Can you work these out from the model? Positions are in its coordinate system, mm. A direction names the side the tool comes from. Round coordinates to 2 decimals unless told otherwise and drop trailing zeros. Write each loop counter-clockwise with the first axis right and the second up, starting at its lowest first coordinate (ties: lowest second). Pieces come first, ordered by that corner, then holes. Notation, with made-up numbers: (46, 44.5) -> (73, 44.5) arc R12 ccw to (73, 65.5) -> close; hole circle Ø10 at (26.25, 47). An arc over 180 degrees is marked (long way). Write item = value, one per line. Start each with the question number.
1) Imagine slicing it at A-A, the plane z = 9.25. Please give me the cut outline in (x, y).
2) Imagine slicing it at B-B, the plane x = -7.5. Please give me the cut outline in (y, z).
3) Thinking about a two-plate mould opening in Y: for faces 1 (the face through (-11.356, -23.102, 3.143)), 2 (the face through (-14.274, 0.628, 5.899)), 3 (the face through (9.23, -0.57, 13.11)), 4 (the face through (11, 6, 6.35)), which applies, +Y half, -Y half, draft (parallel to the pull), parting line (faces both ways), or undercut?
4) I'm going to push flat-ended pins straight in: pin 1 (6.5 mm diameter, centred on x = 23.81, y = 0, fed in from -Z); pin 2 (8 mm diameter, centred on y = -1.5, z = 9.5, fed in from +X); pin 3 (23 mm diameter, centred on x = 1.5, y = 3.5, fed in from +Z); pin 4 (1 mm diameter, centred on x = -14.5, y = 0.5, fed in from +Z). Where does each tip first touch, or does it pass through?
5) Imagine slicing it at C-C, the plane y = -19.5. Please give me the cut outline in (x, z).
6) If I drill on line 1 (Z direction, x = 0, y = -21); line 2 (Y direction, x = -4.5, z = 10.5); line 3 (X direction, y = 3.5, z = 1), over which ranges is the centre line in solid material (lowest first)?
7) Imagine slicing it at D-D, the plane z = 4. State how many separate pieces and enclosed holes the cut face has, then the cut area to 3 significant figures.
8) For faces 5 (the face through (-13, 7, 5.461)), 6 (the face through (-7, 0, 0)), 7 (the face through (-5, 5, 25.4)), 8 (the face through (-6.35, -1, 13)), 9 (the face through (-14.274, 0.628, 0.438)), which set-ups out of +Z, -Z, +X, -X, +Y, -Y let a thin tool reach every point of the face, with its end or its side?
from build123d import *

# Parameters (mm, degrees)
SKETCH1_R              = 14.2875
BOSS_EXTRUDE1_DEPTH    = 0.889
SKETCH2_R              = 28.575
BOSS_EXTRUDE2_DEPTH    = 4.572
SKETCH3_R              = 14.2875
BOSS_EXTRUDE3_DEPTH    = 0.889
SKETCH4_R              = 12.192
BOSS_EXTRUDE4_DEPTH    = 19.05
SKETCH5_R              = 2.54
CUT_EXTRUDE1_DEPTH     = 48.2636263
CUT_EXTRUDE2_DEPTH     = 48.730716001
F_10_24_TAPPED_HOLE1_D = 3.7973
CIRPATTERN1_COUNT      = 2
CIRPATTERN1_ANGLE      = 90


with BuildPart() as part:
    # Sketch1 → Boss-Extrude1 (new body)
    with BuildSketch(Plane.XY):
        Circle(SKETCH1_R)
    extrude(amount=BOSS_EXTRUDE1_DEPTH)

    # Sketch2 → Boss-Extrude2 (add)
    with BuildSketch(Plane.XY.offset(0.889)):
        Circle(SKETCH2_R)
    extrude(amount=BOSS_EXTRUDE2_DEPTH)

    # Sketch3 → Boss-Extrude3 (add)
    with BuildSketch(Plane.XY.offset(5.461)):
        Circle(SKETCH3_R)
    extrude(amount=BOSS_EXTRUDE3_DEPTH)

    # Sketch4 → Boss-Extrude4 (add)
    with BuildSketch(Plane.XY.offset(6.35)):
        with Locations(Location((0, 0, 0), (0, 0, 180))):
            Circle(SKETCH4_R)
    extrude(amount=BOSS_EXTRUDE4_DEPTH)

    # Sketch5 → Cut-Extrude1 (cut, through all)
    with BuildSketch(Plane(origin=(0, 0, 0.889), x_dir=(-1, 0, 0), z_dir=(0, 0, -1))):
        with Locations((-11.90625, 20.622229928)):
            Circle(SKETCH5_R)
        with Locations((11.90625, 20.622229928)):
            Circle(SKETCH5_R)
        with Locations((23.8125, 0)):
            Circle(SKETCH5_R)
        with Locations((11.90625, -20.622229928)):
            Circle(SKETCH5_R)
        with Locations((-11.90625, -20.622229928)):
            Circle(SKETCH5_R)
        with Locations((-23.8125, 0)):
            Circle(SKETCH5_R)
    extrude(amount=-CUT_EXTRUDE1_DEPTH, mode=Mode.SUBTRACT)

    # Sketch6 → Cut-Extrude2 (cut, through all)
    with BuildSketch(Plane.XY.offset(25.4)):
        Polygon((0, 7.332348419), (-6.35, 3.666174209), (-6.35, -3.666174209), (0, -7.332348419), (6.35, -3.666174209), (6.35, 3.666174209), align=None)
    extrude(amount=-CUT_EXTRUDE2_DEPTH, mode=Mode.SUBTRACT)

    # #10-24 Tapped Hole1 (through all)
    with Locations(Plane(origin=(12.192, 0, 14.9225), x_dir=(0, 0, 1), z_dir=(1, 0, 0))):
        with Locations((0, 0)):
            f_10_24_tapped_hole1 = Hole(F_10_24_TAPPED_HOLE1_D / 2)

    # CirPattern1: #10-24 Tapped Hole1 ×2 about axis
    cirpattern1_axis = Axis((0, 0, 5.461), (0, 0, 1))
    for i in range(1, CIRPATTERN1_COUNT):
        add(f_10_24_tapped_hole1.rotate(cirpattern1_axis, i * CIRPATTERN1_ANGLE / (CIRPATTERN1_COUNT - 1)), mode=Mode.SUBTRACT)


solid = part.part
Reported:
q1.outline = circle Ø24.38 at (0, 0); hole (-6.35, -3.67) -> (0, -7.33) -> (6.35, -3.67) -> (6.35, 3.67) -> (0, 7.33) -> (-6.35, 3.67) -> close
q2.outline = (-27.57, 0.89) -> (-12.16, 0.89) -> (-12.16, 0) -> (12.16, 0) -> (12.16, 0.89) -> (27.57, 0.89) -> (27.57, 5.46) -> (12.16, 5.46) -> (12.16, 6.35) -> (9.61, 6.35) -> (9.61, 25.4) -> (-9.61, 25.4) -> (-9.61, 6.35) -> (-12.16, 6.35) -> (-12.16, 5.46) -> (-27.57, 5.46) -> close; hole circle Ø3.8 at (0, 14.92)
q3.face_1 = undercut
q3.face_2 = parting line
q3.face_3 = undercut
q3.face_4 = draft
q4.pin_1 = 0.89
q4.pin_2 = 14.29
q4.pin_3 = 25.4
q4.pin_4 = 6.35
q5.outline = (-20.89, 0.89) -> (-14.18, 0.89) -> (-14.18, 5.46) -> (-20.89, 5.46) -> close; (-9.63, 0.89) -> (9.63, 0.89) -> (9.63, 5.46) -> (-9.63, 5.46) -> close; (14.18, 0.89) -> (20.89, 0.89) -> (20.89, 5.46) -> (14.18, 5.46) -> close
q6.line_1 = 0.89 to 5.46
q6.line_2 = -11.33 to -4.73, 4.73 to 11.33
q6.line_3 = -28.36 to -6.35, 6.35 to 28.36
q7.separate_pieces = 1
q7.enclosed_holes = 7
q7.area = 2,300 mm²
q8.face_5 = +Z
q8.face_6 = -Z, +X, -X, +Y, -Y
q8.face_7 = +Z, +X, -X, +Y, -Y
q8.face_8 = +Z, -Z
q8.face_9 = -Z
